Can you work these out from the model? Positions are in its coordinate system, mm. Face numbers are marked on the shaded views. A direction names the side the tool comes from. Give positions to 0.01 mm unless a question says otherwise; leave off trailing zeros. Loops run counter-clockwise (first coordinate to the right, second up) from the corner with the lowest first, then second, coordinate; pieces in that order, holes last. Notation, with made-up numbers: (82.25, 78.25) - (131.25, 78.25) arc R33 ccw to (131.25, 113.25) - close; hole circle Ø9 at (31.25, -9). An arc over 180 degrees is marked (long way). Use a Markdown table: item, result. Add a question column.
```python
from build123d import *

# Parameters (mm, degrees)
BOSS_EXTRUDE1_DEPTH             = 35
BOSS_EXTRUDE4_REACH             = 109.487
SKETCH4_R                       = 17.5
BOSS_EXTRUDE4_DIRECTION_2_REACH = 109.487
BOSS_EXTRUDE3_DEPTH             = 36
BOSS_EXTRUDE3_DEPTH_BACK        = 35
SKETCH3_R                       = 17.5


with BuildPart() as part:
    # Sketch1 → Boss-Extrude1 (new body)
    with BuildSketch(Plane(origin=(0, 0, 0), x_dir=(1, 0, 0), z_dir=(0, 1, 0))):
        Polygon((0, -90), (82.692132723, -90), (82.692132723, 55), (47.206666819, 55), (47.206666819, -55), (0, -55), align=None)
    extrude(amount=BOSS_EXTRUDE1_DEPTH)


with BuildPart() as body_2:

    # Boss-Extrude4: up to this face of the body (flat: up to its plane)
    boss_extrude4_end = Plane(part.part.faces().sort_by_distance((0, 17.5, 72.5))[0])
    # Sketch4 → Boss-Extrude4 (new, up to the picked face)
    with BuildSketch(Plane.ZY.offset(-47.206666819), mode=Mode.PRIVATE) as boss_extrude4_sk1:
        with Locations(Location((-55, 17.5, 0), (0, 0, 180))):
            Circle(SKETCH4_R)
    boss_extrude4_tool1 = split(extrude(boss_extrude4_sk1.sketch, amount=BOSS_EXTRUDE4_REACH, mode=Mode.PRIVATE), bisect_by=boss_extrude4_end, keep=Keep.BOTH, mode=Mode.PRIVATE)
    add(boss_extrude4_tool1.solids().sort_by(Axis((47.206667, 17.5, -55), (-1, 0, 0)))[0])


    # Boss-Extrude4 direction 2: up to this face of the body (flat: up to its plane)
    boss_extrude4_direction_2_end = Plane(part.part.faces().sort_by_distance((82.692132723, 17.5, 17.5))[0])
    # Sketch4 → Boss-Extrude4 direction 2 (add, up to the picked face)
    with BuildSketch(Plane.ZY.offset(-47.206666819), mode=Mode.PRIVATE) as boss_extrude4_direction_2_sk1:
        with Locations(Location((-55, 17.5, 0), (0, 0, 180))):
            Circle(SKETCH4_R)
    boss_extrude4_direction_2_tool1 = split(extrude(boss_extrude4_direction_2_sk1.sketch, amount=-BOSS_EXTRUDE4_DIRECTION_2_REACH, mode=Mode.PRIVATE), bisect_by=boss_extrude4_direction_2_end, keep=Keep.BOTH, mode=Mode.PRIVATE)
    add(boss_extrude4_direction_2_tool1.solids().sort_by(Axis((47.206667, 17.5, -55), (1, 0, 0)))[0])


with BuildPart() as body_3:
    # Sketch3 → Boss-Extrude3 (new, two sides: drawn at the far end of the back side and taken through both)
    with BuildSketch(Plane.XY.offset(90).offset(-BOSS_EXTRUDE3_DEPTH_BACK)):
        with Locations((0, 17.5)):
            Circle(SKETCH3_R)
    extrude(amount=BOSS_EXTRUDE3_DEPTH + BOSS_EXTRUDE3_DEPTH_BACK)

    # Combine1: union part, body 2
    add(part.part)
    add(body_2.part)


solid = body_3.part
```
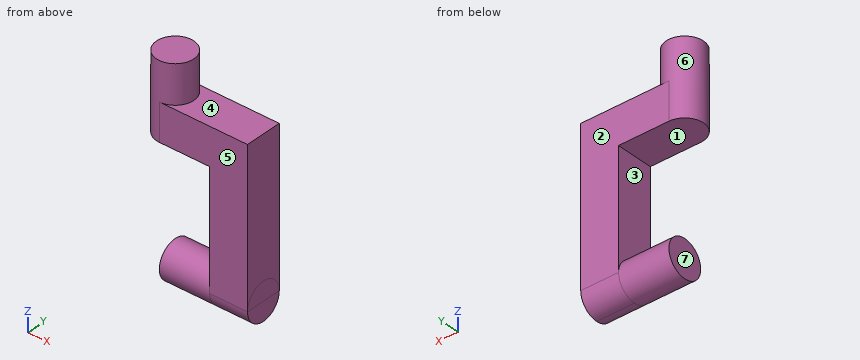
1. Will these pins go through, and if not, where does the flat tip stop? P1, Ø12, axis at y = 30, z = 105.5, coming from the +X side; P2, Ø2, axis at x = 12.5, y = 13, coming from the -Z side; P3, Ø10.5, axis at y = 19, z = -54.5, coming from the -X side.
2. Suppose I cut it at A-A (y = 4.5). List the corners of the cut face in (x, z) for me, and give its area (3 significant figures).
3. If we mould it in two halves opening along Z, with no side actions, what happens to the marked faces 1, 2, 3 and 4? For each: released by +Z, released by -Z, zero draft, split by the parting line, or undercut.
4. Please list where these lines run through material, in increasing order: line 1 along X through (y, z) = (19, 41.5); line 2 along Z through (x, y) = (42.5, 13); line 3 along Z through (x, y) = (38.5, 27.5). Write a range as [from, to].
5. On a 3-axis mill with a long thin cutter (end or side, diameter ignored), from which of +Z, -Z, +X, -X, +Y, -Y can I reach the whole of each face in a straight line? I mean the marked faces 5, 6 and 7. Say none if no direction works.
6. Suppose I cut it at C-C (z = 22). List the corners of the cut face in (x, y) for me, and give its area (3 significant figures).
7. Suppose I cut it at D-D (x = 69). List the corners of the cut face in (y, z) for me, and give its area (3 significant figures).
8. Suppose I cut it at B-B (x = 6.5). List the corners of the cut face in (y, z) for me, and give its area (3 significant figures).
Results below:
| question | item | result |
|---|---|---|
| 1 | P1 | x = 16.25 |
| 1 | P2 | z = -72.15 |
| 1 | P3 | x = 0 |
| 2 | outline | (-11.72, 55) - (47.21, 55) - (47.21, -43.28) - (0, -43.28) - (0, -66.72) - (82.69, -66.72) - (82.69, 90) - (11.72, 90) - (11.72, 126) - (-11.72, 126) - close |
| 2 | area | 9,570 mm² |
| 3 | face 1 | undercut |
| 3 | face 2 | zero draft |
| 3 | face 3 | undercut |
| 3 | face 4 | released by +Z |
| 4 | line 1 | [47.21, 82.69] |
| 4 | line 2 | [-71.91, -38.09], [55, 90] |
| 4 | line 3 | [-69.36, -40.64], [55, 90] |
| 5 | face 5 | +Z, -Z, +X, -X, -Y |
| 5 | face 6 | +Z |
| 5 | face 7 | -Z, -X, +Y, -Y |
| 6 | outline | (47.21, 0) - (82.69, 0) - (82.69, 35) - (47.21, 35) - close |
| 6 | area | 1,240 mm² |
| 7 | outline | (0, -55) arc R17.5 ccw to (35, -55) - (35, 90) - (0, 90) - close |
| 7 | area | 5,560 mm² |
| 8 | outline | circle Ø35 at (17.5, -55); (0, 55) - (35, 55) - (35, 90) - (33.75, 90) - (33.75, 126) - (1.25, 126) - (1.25, 90) - (0, 90) - close |
| 8 | area | 3,360 mm² |
